Work out the finished part from the listing and answer in its coordinate system (mm). Face numbers are marked on the shaded views. A direction names the side the tool comes from. Coordinates: 2 decimals unless noted, no trailing zeros. Order: outer loops, then holes, each group sorted by start corner. A loop starts at its lowest first (then second) coordinate and runs counter-clockwise, first axis right, second up. Notation, with made-up numbers: M 65,76.5 L 77,76.5 A24 cw 77,107.5 Z; hole C 78,-37 d10. An arc over 180 degrees is marked long. Answer in a Markdown table with one row per item. Add a question column.
Item 1: The mould has two halves that part along X. Classify the marked faces 1, 2, 3 and 4: released by +X, released by -X, zero draft, split by the parting line, or undercut.
Item 2: The part is cut by section C-C (z = -5.5). Write down the section's boundary in (x, y).
Item 3: The part is cut by section A-A (x = 0). Write down the section's boundary in (y, z), then the cut area to 3 significant figures.
Item 4: The part is cut by section D-D (z = 1.5). Write down the section's boundary in (x, y), then the cut area to 3 significant figures.
Item 5: The part is cut by section B-B (y = 4.75). Write down the section's boundary in (x, z), then the cut area to 3 significant figures.
Item 6: Which of the six approach directions +Z, -Z, +X, -X, +Y, -Y give full straight-line access (tool end or side, diameter ignored) to the marked faces 5, 6 and 7?
Item 7: Consider line 1 (X direction, y = 9.5, z = 0.5); line 2 (Y direction, x = 0, z = -0.05). Determine where each line is inside the solid, lowest interval first. Write a range as from..to.
Item 8: Flat-ended cylindrical pins translate along their axes: pin 1 Ø3 at (y, z) = (18.5, -1) entering from -X; pin 2 Ø0.9 at (y, z) = (16.5, 0) entering from +X; pin 3 Ø1.7 at (x, y) = (-0.5, 16) entering from -Z. Find the tip coordinate at first contact, or state that the pin passes through.
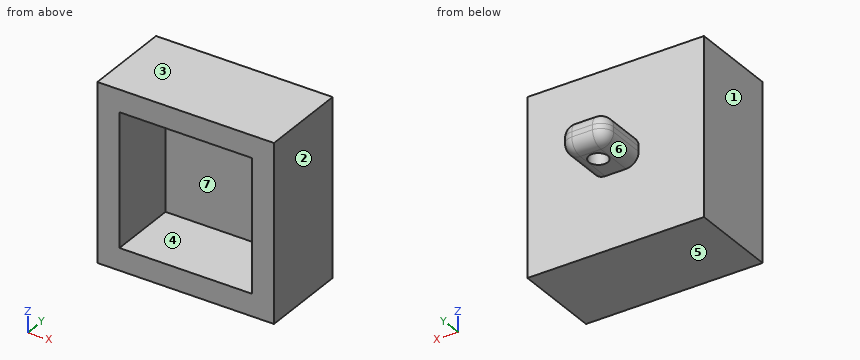
from build123d import *

# Parameters (mm, degrees)
SKETCH1_W           = 28
SKETCH1_H           = 28
SKETCH1_W_2         = 21
SKETCH1_H_2         = 21
BOSS_EXTRUDE1_DEPTH = 11
SKETCH2_W           = 28
SKETCH2_H           = 28
BOSS_EXTRUDE2_DEPTH = 3
SKETCH3_W           = 7.3
SKETCH3_H           = 4.8
BOSS_EXTRUDE3_DEPTH = 8
FILLET3_R           = 2
SKETCH4_R           = 1.5
CUT_EXTRUDE1_DEPTH  = 5


with BuildPart() as part:
    # Sketch1 → Boss-Extrude1 (new body)
    with BuildSketch(Plane(origin=(0, 0, 0), x_dir=(1, 0, 0), z_dir=(0, 1, 0))):
        Rectangle(SKETCH1_W, SKETCH1_H)
        Rectangle(SKETCH1_W_2, SKETCH1_H_2, mode=Mode.SUBTRACT)
    extrude(amount=BOSS_EXTRUDE1_DEPTH)

    # Sketch2 → Boss-Extrude2 (add)
    with BuildSketch(Plane(origin=(0, 11, 0), x_dir=(1, 0, 0), z_dir=(0, 1, 0))):
        Rectangle(SKETCH2_W, SKETCH2_H)
    extrude(amount=BOSS_EXTRUDE2_DEPTH)

    # Sketch3 → Boss-Extrude3 (add)
    with BuildSketch(Plane(origin=(0, 14, 0), x_dir=(1, 0, 0), z_dir=(0, 1, 0))):
        Rectangle(SKETCH3_W, SKETCH3_H)
    extrude(amount=BOSS_EXTRUDE3_DEPTH)

    # Fillet3
    fillet3_edges = [part.edges().sort_by_distance(p)[0] for p in [
        (-3.65, 18, -2.4),
        (-3.65, 18, 2.4),
        (3.65, 18, 2.4),
        (3.65, 18, -2.4),
        (-3.65, 22, 0),
        (0, 22, 2.4),
        (3.65, 22, 0),
        (0, 22, -2.4),
    ]]
    fillet(fillet3_edges, radius=FILLET3_R)

    # Sketch4 → Cut-Extrude1 (cut)
    with BuildSketch(Plane(origin=(0, 0, -2.4), x_dir=(-1, 0, 0), z_dir=(0, 0, -1))):
        with Locations((0, 18.128577291)):
            Circle(SKETCH4_R)
    extrude(amount=-CUT_EXTRUDE1_DEPTH, mode=Mode.SUBTRACT)


solid = part.part
Reply:
| question | item | result |
|---|---|---|
| 1 | face 1 | released by -X |
| 1 | face 2 | released by +X |
| 1 | face 3 | zero draft |
| 1 | face 4 | undercut |
| 2 | outline | M -14,0 L -10.5,0 L -10.5,11 L 10.5,11 L 10.5,0 L 14,0 L 14,14 L -14,14 Z |
| 3 | outline | M 0,-14 L 14,-14 L 14,-2.4 L 16.63,-2.4 L 16.63,2.4 L 14,2.4 L 14,14 L 0,14 L 0,10.5 L 11,10.5 L 11,-10.5 L 0,-10.5 Z; M 19.63,-2.4 L 20,-2.4 A2 ccw 22,-0.4 L 22,0.4 A2 ccw 20,2.4 L 19.63,2.4 Z |
| 3 | area | 183 mm2 |
| 4 | outline | M -14,0 L -10.5,0 L -10.5,11 L 10.5,11 L 10.5,0 L 14,0 L 14,14 L 3.32,14 L 3.32,20 A1.67 ccw 1.65,21.67 L -1.65,21.67 A1.67 ccw -3.32,20 L -3.32,14 L -14,14 Z; hole C 0,18.13 d3 |
| 4 | area | 204 mm2 |
| 5 | outline | M -14,-14 L 14,-14 L 14,14 L -14,14 Z; hole M -10.5,-10.5 L 10.5,-10.5 L 10.5,10.5 L -10.5,10.5 Z |
| 5 | area | 343 mm2 |
| 6 | face 5 | -Z, +X, -X, +Y, -Y |
| 6 | face 6 | -Z, -X, +Y |
| 6 | face 7 | -Y |
| 7 | line 1 | x = -14..-10.5, 10.5..14 |
| 7 | line 2 | y = 11..16.63, 19.63..22 |
| 8 | pin 1 | stops at x = -3.65 |
| 8 | pin 2 | stops at x = 3.65 |
| 8 | pin 3 | stops at z = -2.4 |
